Model file for the job. Use its own axes, mm. A direction names the side the tool comes from. Coordinates: 2 decimals unless noted, no trailing zeros. Write each loop counter-clockwise with the first axis right and the second up, starting at its lowest first coordinate (ties: lowest second). Pieces come first, ordered by that corner, then holes.
Q1. Drill centre lines: probe 1 along X at (y, z) = (-1.9, 1.4); probe 2 along Z at (x, y) = (-54, -0.4). Where is each one in solid material? Low to high.
Q2. Which spindle directions (+Z, -Z, +X, -X, +Y, -Y) get a long thin tool onto all of the face, cutting with end or side? Do faces 1 (the flat face through (89, 0, 0)), 2 (the flat face through (-89, 0, 0)), 3 (the cylindrical face through (-1.279, 2.374, -0.748)). Say none if no direction does.
Q3. Pin check, flat tips, straight feed: P1, Ø0.7, axis at y = -1, z = 0.5, coming from the +X side; P2, Ø1.5, axis at x = 88, z = 0, coming from the -Y side; P3, Ø0.7, axis at y = -1.5, z = 1, coming from the -X side; P4, Ø1, axis at x = -66, z = 0.5, coming from the +Y side. Stop position of each tip, or through.
Q4. Band-saw the part on B-B, the plane x = -42. Write the cut outline in (y, z).
Q5. Band-saw the part on C-C, the plane y = 1.1. Write the cut outline in (x, z), plus the area to 3 significant figures.
Q6. Band-saw the part on A-A, the plane z = 0. Write the cut outline in (x, y).
Solid Edge part; units mm, degrees
sketch "Sketch1" plane through (0, 0, 0) normal (1, 0, 0) x (0, 1, 0)
  circle A0 centre (0, 0) radius 2.4892
extrude "Protrusion1" add sketch "Sketch1" along normal mid plane 182.7784
sketch "Sketch2" plane through (0, -2.4892, 0) normal (0, -1, 0) x (1, 0, 0)
  line L0 (91.3892, 2.4892) -> (91.3892, -2.4892)
  line L1 (91.3892, -2.4892) -> (86.4092, -2.4892)
  line L2 (86.4092, -2.4892) -> (86.4092, 2.4892)
  line L3 (86.4092, 2.4892) -> (91.3892, 2.4892)
extrude "ExtrudedCutout_1" cut sketch "Sketch2" against normal blind 2.4892
mirror "Mirror1" about plane through (0, 0, 0) normal (1, 0, 0) of "ExtrudedCutout_1"
properties material "Wood, Pine"
Answer sheet:
1. probe 1: x = -86.41 to 86.41
1. probe 2: z = -2.46 to 2.46
2. face 1: +Z, -Z, +X, -Y
2. face 2: +Z, -Z, -X, -Y
2. face 3: +X, -X
3. P1: stops at x = 86.41
3. P2: stops at y = 0
3. P3: stops at x = -86.41
3. P4: stops at y = 2.49
4. outline: circle Ø4.98 at (0, 0)
5. outline: (-91.39, -2.23) - (91.39, -2.23) - (91.39, 2.23) - (-91.39, 2.23) - close
5. area: 816 mm2
6. outline: (-91.39, 0) - (-86.41, 0) - (-86.41, -2.49) - (86.41, -2.49) - (86.41, 0) - (91.39, 0) - (91.39, 2.49) - (-91.39, 2.49) - close
